from build123d import *

# Parameters (mm, degrees)
F3_DEPTH = 2.701


with BuildPart() as f1:
    # F0 (on Right) → F1 (revolve)
    with BuildSketch(Plane.YZ):
        Polygon((0, 23), (0, 8.5), (2.5, 8.5), (2.5, 23), (2.7, 23), (2.7, 27.5), (0.2, 27.5), (0.2, 23), align=None)
    revolve(axis=Axis((0, 1.25, 0), (0, 1, 0)))

    # F2 (on Front) → F3 (cut, through all)
    with BuildSketch(Plane.XZ):
        with BuildLine():
            Line((2.75, 10.6), (-2.75, 10.6))
            Line((-2.75, 10.6), (-2.75, 8.042854))
            ThreePointArc((-2.75, 8.042854), (0, 8.5), (2.75, 8.042854))
            Line((2.75, 8.042854), (2.75, 10.6))
        make_face()
    extrude(amount=-F3_DEPTH, mode=Mode.SUBTRACT)


solid = f1.part
Geometry check sheet. Reference: the model listing, model coordinates, mm. A direction names the side the tool comes from. Round coordinates to 2 decimals unless told otherwise and drop trailing zeros. Write each loop counter-clockwise with the first axis right and the second up, starting at its lowest first coordinate (ties: lowest second). Pieces come first, ordered by that corner, then holes. Notation, with made-up numbers: (-33.5, 16) -> (23.5, 16) arc R14 ccw to (23.5, 35) -> close; hole circle Ø6 at (77, -8). An arc over 180 degrees is marked (long way). One line per item, written item: value. Start each with the question number.
(1) Cross-section at D-D, the plane x = 11. Record the cut outline in (y, z), and give its area (3 significant figures).
(2) Cross-section at B-B, the plane x = 0. Record the cut outline in (y, z), and give its area (4 significant figures).
(3) Access from +Z, -Z, +X, -X, +Y, -Y to the whole of each face (thin tool, end or side, straight path). Record for faces 1 (the flat face through (-18.2, 2.7, 14.4)), 2 (the flat face through (0, 2.5, -10)), 3 (the flat face through (0, 1, 10.6)).
(4) Go/stop test with flat-tipped pins: pin 1 Ø6 at (x, z) = (-18.5, 4) entering from +Y; pin 2 Ø1.2 at (y, z) = (1.5, 9) entering from -X; pin 3 Ø10 at (x, z) = (0, 0) entering from +Y; pin 4 Ø0.8 at (y, z) = (1, 10) entering from +X. Record where each tip stops, or that it passes through.
(5) Cross-section at C-C, the plane y = 1.2. Record the cut outline in (x, z), and give its area (3 significant figures).
(6) Draft check along Z on faces 4 (the cylindrical face through (0.335, 1.268, -8.493)), 5 (the flat face through (-18.2, 0.2, -14.4)), 6 (the cylindrical face through (-26.846, 1.432, -5.961)). Enter one of: +Z half, -Z half, draft (parallel to the pull), parting line (faces both ways), or undercut.
(7) Scan lines: line 1 (Z direction, x = 0.5, y = 0.65); line 2 (X direction, y = 2.6, z = 0); line 3 (X direction, y = 1.65, z = 0). Record each from-to range of solid material in increasing order. Write a range as [from, to].
(8) Cross-section at A-A, the plane z = 0. Record the cut outline in (x, y).
Answer:
1. outline: (0, -20.2) -> (0.2, -20.2) -> (0.2, -25.2) -> (2.7, -25.2) -> (2.7, -20.2) -> (2.5, -20.2) -> (2.5, 20.2) -> (2.7, 20.2) -> (2.7, 25.2) -> (0.2, 25.2) -> (0.2, 20.2) -> (0, 20.2) -> close
1. area: 126 mm²
2. outline: (0, -23) -> (0.2, -23) -> (0.2, -27.5) -> (2.7, -27.5) -> (2.7, -23) -> (2.5, -23) -> (2.5, -8.5) -> (0, -8.5) -> close; (0, 10.6) -> (2.5, 10.6) -> (2.5, 23) -> (2.7, 23) -> (2.7, 27.5) -> (0.2, 27.5) -> (0.2, 23) -> (0, 23) -> close
2. area: 89.75 mm²
3. face 1: +Z, -Z, +X, -X, +Y
3. face 2: +Y
3. face 3: +Y, -Y
4. pin 1: y = 2.5
4. pin 2: x = -26.19
4. pin 3: through
4. pin 4: x = 25.77
5. outline: circle Ø55 at (0, 0); hole (-2.75, 8.04) arc R8.5 ccw (long way) to (2.75, 8.04) -> (2.75, 10.6) -> (-2.75, 10.6) -> close
5. area: 2,140 mm²
6. face 4: undercut
6. face 5: draft
6. face 6: parting line
7. line 1: [-27.5, -8.49], [10.6, 27.5]
7. line 2: [-27.5, -23], [23, 27.5]
7. line 3: [-27.5, -8.5], [8.5, 27.5]
8. outline: (-27.5, 0.2) -> (-23, 0.2) -> (-23, 0) -> (-8.5, 0) -> (-8.5, 2.5) -> (-23, 2.5) -> (-23, 2.7) -> (-27.5, 2.7) -> close; (8.5, 0) -> (23, 0) -> (23, 0.2) -> (27.5, 0.2) -> (27.5, 2.7) -> (23, 2.7) -> (23, 2.5) -> (8.5, 2.5) -> close
